Here's how the part is built. I have some questions about the finished solid (model axes, mm). A direction names the side the tool comes from. Give positions to 0.01 mm unless a question says otherwise; leave off trailing zeros. Use a Markdown table: item, result.
from build123d import *

# Parameters (mm, degrees)
SKIZZE1_W                                            = 220
SKIZZE1_H                                            = 220
AUFSATZ_LINEAR_AUSTRAGEN1_DEPTH                      = 15
F_6_0MM_STIFTLOCH1_D                                 = 6
F_5_0MM_STIFTLOCH1_D                                 = 5
M5_GEWINDEBOHRUNG1_D                                 = 4.2
STIRNSENKUNG_F_R_M6_ZYLINDERSCHRAUBE_MIT_D           = 6.6
STIRNSENKUNG_F_R_M6_ZYLINDERSCHRAUBE_MIT_CBORE_D     = 11
STIRNSENKUNG_F_R_M6_ZYLINDERSCHRAUBE_MIT_CBORE_DEPTH = 4.4
M4_GEWINDEBOHRUNG1_D                                 = 3.3
M4_GEWINDEBOHRUNG1_DEPTH                             = 11.5
M4_GEWINDEBOHRUNG1_TIP                               = 0.991420021
STIRNSENKUNG_F_R_M5_SECHSKANTSCHRAUBE_MI_D           = 5.3
STIRNSENKUNG_F_R_M5_SECHSKANTSCHRAUBE_MI_CBORE_D     = 10
STIRNSENKUNG_F_R_M5_SECHSKANTSCHRAUBE_MI_CBORE_DEPTH = 5.4
STIRNSENKUNG_F_R_M6_ZYLINDERSCHRAUBE_2_D             = 6.6
STIRNSENKUNG_F_R_M6_ZYLINDERSCHRAUBE_2_CBORE_D       = 11
STIRNSENKUNG_F_R_M6_ZYLINDERSCHRAUBE_2_CBORE_DEPTH   = 4.4
F_4_0MM_STIFTLOCH1_D                                 = 4


with BuildPart() as part:
    # Skizze1 → Aufsatz-Linear austragen1 (new body)
    with BuildSketch(Plane(origin=(0, 0, 0), x_dir=(-1, 0, 0), z_dir=(0, 0, -1))):
        Rectangle(SKIZZE1_W, SKIZZE1_H)
    extrude(amount=-AUFSATZ_LINEAR_AUSTRAGEN1_DEPTH)

    # Ø6.0mm Stiftloch1 (through all)
    with Locations(Plane(origin=(0, 0, 0), x_dir=(-1, 0, 0), z_dir=(0, 0, -1))):
        with Locations((-100, -80), (-100, 80), (100, 80), (100, -80)):
            Hole(F_6_0MM_STIFTLOCH1_D / 2)

    # Ø5.0mm Stiftloch1 (through all)
    with Locations(Plane(origin=(0, 0, 0), x_dir=(-1, 0, 0), z_dir=(0, 0, -1))):
        with Locations((0, 50), (0, -50), (105, -65), (85, -65), (-85, -65), (-105, -65)):
            Hole(F_5_0MM_STIFTLOCH1_D / 2)

    # M5 Gewindebohrung1 (through all)
    with Locations(Plane.XY.offset(15)):
        with Locations((-25, 50), (25, 50), (25, -50), (-25, -50)):
            Hole(M5_GEWINDEBOHRUNG1_D / 2)

    # Stirnsenkung f_r M6 Zylinderschraube mit (through all)
    with Locations(Plane.XY.offset(15)):
        with Locations((100, -100), (100, 0), (-100, -100), (-100, 0), (-100, 100), (100, 100)):
            CounterBoreHole(STIRNSENKUNG_F_R_M6_ZYLINDERSCHRAUBE_MIT_D / 2, STIRNSENKUNG_F_R_M6_ZYLINDERSCHRAUBE_MIT_CBORE_D / 2, STIRNSENKUNG_F_R_M6_ZYLINDERSCHRAUBE_MIT_CBORE_DEPTH)

    # M4 Gewindebohrung1
    with Locations(Plane.XY.offset(15)):
        with Locations((-56, 54), (-56, 36), (-56, -36), (-56, -54), (9, -76), (-9, -76)):
            Hole(M4_GEWINDEBOHRUNG1_D / 2, depth=M4_GEWINDEBOHRUNG1_DEPTH)
            with Locations((0, 0, -(M4_GEWINDEBOHRUNG1_DEPTH + M4_GEWINDEBOHRUNG1_TIP / 2))):  # 118° drill point
                Cone(0, M4_GEWINDEBOHRUNG1_D / 2, M4_GEWINDEBOHRUNG1_TIP, mode=Mode.SUBTRACT)

    # Stirnsenkung für M5 Sechskantschraube mit Schaft1 (through all)
    with Locations(Plane(origin=(0, 0, 0), x_dir=(-1, 0, 0), z_dir=(0, 0, -1))):
        with Locations((95, -57.5), (95, -72.5), (-95, -57.5), (-95, -72.5)):
            CounterBoreHole(STIRNSENKUNG_F_R_M5_SECHSKANTSCHRAUBE_MI_D / 2, STIRNSENKUNG_F_R_M5_SECHSKANTSCHRAUBE_MI_CBORE_D / 2, STIRNSENKUNG_F_R_M5_SECHSKANTSCHRAUBE_MI_CBORE_DEPTH)

    # Stirnsenkung f_r M6 Zylinderschraube 2 (through all)
    with Locations(Plane(origin=(0, 0, 0), x_dir=(-1, 0, 0), z_dir=(0, 0, -1))):
        with Locations((-80, 102.5), (-80, 77.5), (80, 77.5), (80, 102.5), (80, -77.5), (80, -102.5), (-80, -77.5), (-80, -102.5)):
            CounterBoreHole(STIRNSENKUNG_F_R_M6_ZYLINDERSCHRAUBE_2_D / 2, STIRNSENKUNG_F_R_M6_ZYLINDERSCHRAUBE_2_CBORE_D / 2, STIRNSENKUNG_F_R_M6_ZYLINDERSCHRAUBE_2_CBORE_DEPTH)

    # Ø4.0mm Stiftloch1 (through all)
    with Locations(Plane(origin=(0, 0, 0), x_dir=(-1, 0, 0), z_dir=(0, 0, -1))):
        with Locations((-100, 90), (-80, 90), (80, 90), (100, 90), (100, -90), (80, -90), (-80, -90), (-100, -90)):
            Hole(F_4_0MM_STIFTLOCH1_D / 2)


solid = part.part
(1) If I drill on line 1 (Y direction, x = -95, z = 4.05); line 2 (Y direction, x = -77, z = 4); line 3 (X direction, y = -78, z = 9.75), over which ranges is the centre line in solid material (lowest first)?
A:
| item | result |
|---|---|
| line 1 | -110 to -77.5, -67.5 to -62.5, -52.5 to 110 |
| line 2 | -110 to -107.11, -97.89 to -82.11, -72.89 to 72.89, 82.11 to 97.89, 107.11 to 110 |
| line 3 | -110 to -102.24, -97.76 to -83.26, -76.74 to 76.74, 83.26 to 97.76, 102.24 to 110 |
(2) Will these pins go through, and if not, where does the flat tip stop? pin 1 (10 mm diameter, centred on x = 100, y = -100, fed in from +Z); pin 2 (2 mm diameter, centred on x = -56, y = 36, fed in from +Z); pin 3 (10 mm diameter, centred on x = 80, y = 102.5, fed in from -Z).
A:
| item | result |
|---|---|
| pin 1 | z = 10.6 |
| pin 2 | z = 3.11 |
| pin 3 | z = 4.4 |
(3) On a 3-axis mill with a long thin cutter (end or side, diameter ignored), from which of +Z, -Z, +X, -X, +Y, -Y can I reach the whole of each face in a straight line? I mean faces 1 (the face through (-96, 100, 10.6)), 2 (the face through (-82.43, 104.73, 9.77)), 3 (the face through (76, 78, 4.4)). Say none if no direction works.
A:
| item | result |
|---|---|
| face 1 | +Z |
| face 2 | +Z, -Z |
| face 3 | -Z |
